Model file for the job. Use its own axes, mm. Coordinates: 2 decimals unless noted, no trailing zeros. Write each loop counter-clockwise with the first axis right and the second up, starting at its lowest first coordinate (ties: lowest second). Pieces come first, ordered by that corner, then holes.
Q1. Band-saw the part on D-D, the plane z = 18. Write the cut outline in (x, y), plus the area to 3 significant figures.
Q2. Band-saw the part on A-A, the plane y = 0. Write the cut outline in (x, z).
Q3. Pin check, flat tips, straight feed: P1, Ø2, axis at x = 4.5, z = 40, coming from the -Y side; P2, Ø0.6, axis at y = 7, z = 68.5, coming from the +X side; P3, Ø5, axis at y = 5.5, z = 51, coming from the +X side. Stop position of each tip, or through.
Q4. Drill centre lines: probe 1 along Z at (x, y) = (-3, 4.5); probe 2 along Y at (x, z) = (0.75, 34.5). Where is each one in solid material? Low to high.
Q5. Band-saw the part on B-B, the plane x = 0. Write the cut outline in (y, z).
Q6. Band-saw the part on C-C, the plane y = 5.75. Write the cut outline in (x, z).
from build123d import *

# Parameters (mm, degrees)
IZIM1_R                     = 5
Y_KSEKLIK_EKSTR_ZYON1_DEPTH = 70
IZIM2_R                     = 7.5
Y_KSEKLIK_EKSTR_ZYON2_DEPTH = 5
IZIM3_W                     = 3
IZIM3_H                     = 2
Y_KSEKLIK_EKSTR_ZYON3_DEPTH = 8


with BuildPart() as part:
    # Çizim1 → Yükseklik-Ekstrüzyon1 (new body)
    with BuildSketch(Plane.XY):
        Circle(IZIM1_R)
    extrude(amount=Y_KSEKLIK_EKSTR_ZYON1_DEPTH)

    # Çizim2 → Yükseklik-Ekstrüzyon2 (add)
    with BuildSketch(Plane(origin=(0, 0, 0), x_dir=(-1, 0, 0), z_dir=(0, 0, -1))):
        Circle(IZIM2_R)
    extrude(amount=Y_KSEKLIK_EKSTR_ZYON2_DEPTH)

    # Çizim3 → Yükseklik-Ekstrüzyon3 (add)
    with BuildSketch(Plane(origin=(0, 0, 0), x_dir=(1, 0, 0), z_dir=(0, 1, 0))):
        with Locations((0, -69)):
            Rectangle(IZIM3_W, IZIM3_H)
    extrude(amount=Y_KSEKLIK_EKSTR_ZYON3_DEPTH)


solid = part.part
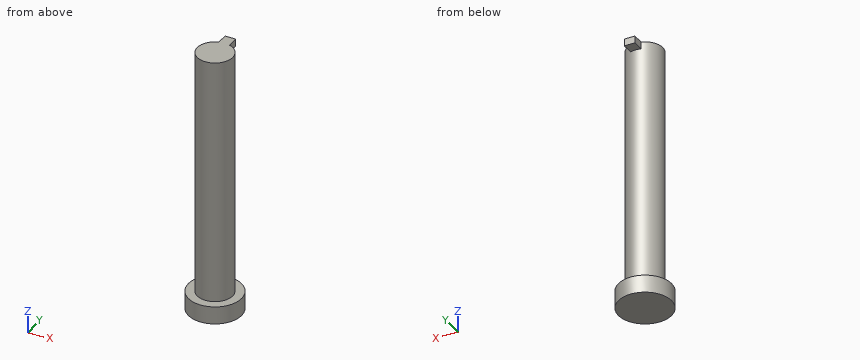
Answer sheet:
1. outline: circle Ø10 at (0, 0)
1. area: 78.5 mm2
2. outline: (-7.5, -5) - (7.5, -5) - (7.5, 0) - (5, 0) - (5, 70) - (-5, 70) - (-5, 0) - (-7.5, 0) - close
3. P1: stops at y = -3.57
3. P2: stops at x = 1.5
3. P3: stops at x = 4
4. probe 1: z = -5 to 0
4. probe 2: y = -4.94 to 4.94
5. outline: (-7.5, -5) - (7.5, -5) - (7.5, 0) - (5, 0) - (5, 68) - (8, 68) - (8, 70) - (-5, 70) - (-5, 0) - (-7.5, 0) - close
6. outline: (-4.82, -5) - (4.82, -5) - (4.82, 0) - (-4.82, 0) - close; (-1.5, 68) - (1.5, 68) - (1.5, 70) - (-1.5, 70) - close
